The drawing under review shows one solid part. Ordinate dimensions are in mm from its lowest x, y, z. Give positions to 0.01 mm unless a question says otherwise; leave off trailing zeros. Loops run counter-clockwise (first coordinate to the right, second up) from the corner with the lowest first, then second, coordinate; pieces in that order, holes last. Notation, with made-up numbers: (34.5, 63.5) - (51.5, 63.5) arc R7 cw to (51.5, 70.5) - close; hole circle Ø10 at (70.5, 79.25). An arc over 180 degrees is marked (long way). Put each result on its own line as item: value. Start each with the question number.
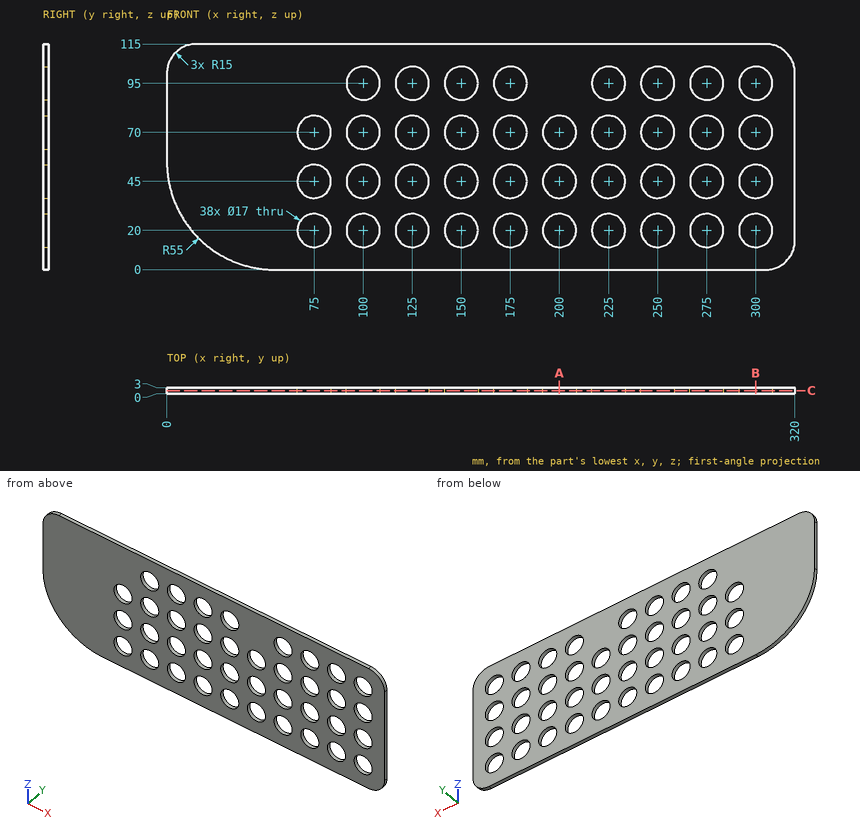
Item 1: Consider section B-B (x = 300). State the section outline as (y, z) points.
Item 2: Consider section A-A (x = 200). State the section outline as (y, z) points.
Item 3: For L1, parallel to Z at x = 300, y = 1.35; L2, parallel to Z at x = 121, y = 0.8, list the stretches that pass through material, from the lowest coordinate up. Write a range as from..to.
Item 4: Consider section C-C (y = 1.55). Count the separate pieces of the cut face and the enclosed holes in it, plus the area to 3 significant figures.
Geometry says:
1. outline: (0, 0) - (3, 0) - (3, 11.5) - (0, 11.5) - close; (0, 28.5) - (3, 28.5) - (3, 36.5) - (0, 36.5) - close; (0, 53.5) - (3, 53.5) - (3, 61.5) - (0, 61.5) - close; (0, 78.5) - (3, 78.5) - (3, 86.5) - (0, 86.5) - close; (0, 103.5) - (3, 103.5) - (3, 115) - (0, 115) - close
2. outline: (0, 0) - (3, 0) - (3, 11.5) - (0, 11.5) - close; (0, 28.5) - (3, 28.5) - (3, 36.5) - (0, 36.5) - close; (0, 53.5) - (3, 53.5) - (3, 61.5) - (0, 61.5) - close; (0, 78.5) - (3, 78.5) - (3, 115) - (0, 115) - close
3. L1: z = 0..11.5, 28.5..36.5, 53.5..61.5, 78.5..86.5, 103.5..115
3. L2: z = 0..12.5, 27.5..37.5, 52.5..62.5, 77.5..87.5, 102.5..115
4. separate pieces: 1
4. enclosed holes: 38
4. area: 27,400 mm2
